Can you work these out from the drawing? Everything is in mm from the part's minimum corner. A direction names the side the tool comes from. Give positions to 0.01 mm unless a question says otherwise; leave off trailing zeros. Write each loop counter-clockwise with the first axis right and the second up, starting at its lowest first coordinate (ties: lowest second). Pieces come first, ordered by that corner, then holes. Notation, with made-up numbers: (30, 27) -> (52, 27) arc R11 cw to (52, 34) -> close; hole circle Ø10 at (86, 62.25). An arc over 180 degrees is marked (long way). Return JSON: item names as keys, results as strings.
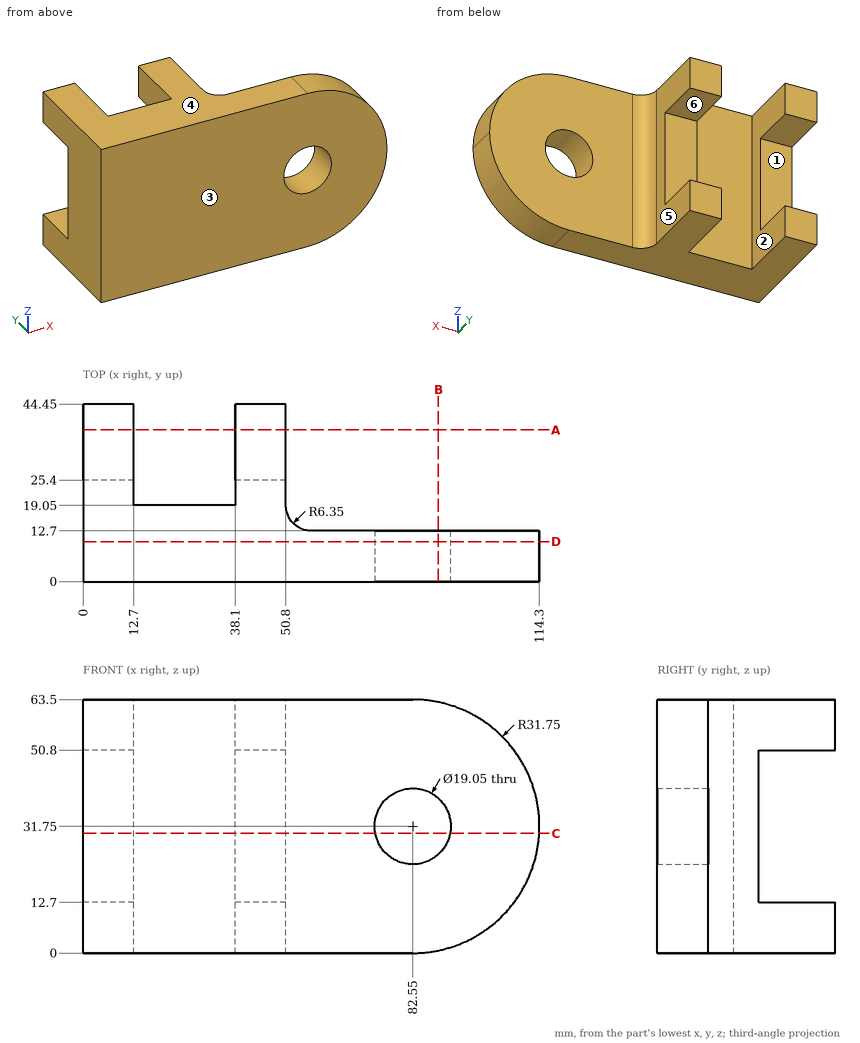
1. Suppose I cut it at D-D, the plane y = 10. List the corners of the cut face in (x, z) for me (3 decimals).
Taken from the geometry:
{"outline": "(0, 0) -> (82.55, 0) arc R31.75 ccw to (114.3, 31.75) arc R31.75 ccw to (82.55, 63.5) -> (0, 63.5) -> close; hole circle Ø19.05 at (82.55, 31.75)"}
2. For pin 1 Ø10 at (x, z) = (41.5, 26) entering from +Y; pin 2 Ø1 at (x, z) = (28.5, 22.5) entering from +Y; pin 3 Ø12.5 at (y, z) = (26, 46) entering from +X; pin 4 Ø5 at (y, z) = (11, 17) entering from -X, each with a flat end and sliding along its axis, tell me the tip position at first contact or that it passes through.
Taken from the geometry:
{"pin 1": "stops at y = 25.4", "pin 2": "stops at y = 19.05", "pin 3": "stops at x = 50.8", "pin 4": "stops at x = 0"}
3. Suppose I cut it at C-C, the plane z = 30. List the corners of the cut face in (x, y) for me.
Taken from the geometry:
{"outline": "(0, 0) -> (73.19, 0) -> (73.19, 12.7) -> (57.15, 12.7) arc R6.35 cw to (50.8, 19.05) -> (50.8, 25.4) -> (38.1, 25.4) -> (38.1, 19.05) -> (12.7, 19.05) -> (12.7, 25.4) -> (0, 25.4) -> close; (91.91, 0) -> (114.25, 0) -> (114.25, 12.7) -> (91.91, 12.7) -> close"}
4. If we mould it in two halves opening along Z, with no side actions, what happens to the marked faces 4, 5 and 6? For each: released by +Z, released by -Z, zero draft, split by the parting line, or undercut.
Taken from the geometry:
{"face 4": "released by +Z", "face 5": "zero draft", "face 6": "undercut"}
5. Suppose I cut it at A-A, the plane y = 38. List the corners of the cut face in (x, z) for me, and give its area (3 significant figures).
Taken from the geometry:
{"outline": "(0, 0) -> (12.7, 0) -> (12.7, 12.7) -> (0, 12.7) -> close; (0, 50.8) -> (12.7, 50.8) -> (12.7, 63.5) -> (0, 63.5) -> close; (38.1, 0) -> (50.8, 0) -> (50.8, 12.7) -> (38.1, 12.7) -> close; (38.1, 50.8) -> (50.8, 50.8) -> (50.8, 63.5) -> (38.1, 63.5) -> close", "area": "645 mm²"}
6. Which directions (+Z, -Z, +X, -X, +Y, -Y) give clear straight access to the entire face, cutting with the end or side of a thin tool? Please do the marked faces 1, 2 and 3.
Taken from the geometry:
{"face 1": "+X, -X, +Y", "face 2": "+Z, -Z, +Y", "face 3": "+Z, -Z, +X, -X, -Y"}
7. Suppose I cut it at B-B, the plane x = 89. List the corners of the cut face in (y, z) for me.
Taken from the geometry:
{"outline": "(0, 0.66) -> (12.7, 0.66) -> (12.7, 24.74) -> (0, 24.74) -> close; (0, 38.76) -> (12.7, 38.76) -> (12.7, 62.84) -> (0, 62.84) -> close"}
8. If I drill on line 1 (X direction, y = 28, z = 57.5); line 2 (Z direction, x = 82.55, y = 6.75) (3 decimals); line 3 (Y direction, x = 92, z = 26.5), over which ranges is the centre line in solid material (lowest first)? Write a range as [from, to].
Taken from the geometry:
{"line 1": "x = [0, 12.7], [38.1, 50.8]", "line 2": "z = [0, 22.225], [41.275, 63.5]", "line 3": "y = [0, 12.7]"}
